Geometry: final body of the model. Coordinates: model frame, mm. A direction names the side the tool comes from. Give positions to 0.01 mm unless a question says otherwise; leave off trailing zeros. Order: outer loops, then holes, each group sorted by start corner. A loop starts at its lowest first (then second) coordinate and runs counter-clockwise, first axis right, second up. Notation, with made-up numbers: (-22.5, -21.5) -> (7.5, -21.5) arc R18 cw to (7.5, -4.5) -> close; hole circle Ø5 at (8, -23.75). An arc over 180 degrees is marked (long way). Answer in a Markdown table with one row per item. Add a question column.
Q1. Cut plane D-D on y = 0.2. Return the cut outline in (x, z) (3 decimals), and give its area (3 significant figures).
Q2. Set-up query: faces 4 (the face through (2.625, 2, -8)), 5 (the face through (4, 1, 0)), 6 (the face through (4, 2, -5.97)), 7 (the face through (4, 2, -9.27)), 8 (the face through (0, 1, -7)). Return all of +Z, -Z, +X, -X, +Y, -Y with unobstructed straight access to the full face (end or side cutting, diameter ignored); none if empty.
Q3. Contact query for flat-ended pins moving along their axis: P1, Ø0.6, axis at y = 2.5, z = -8, coming from the -X side (3 decimals); P2, Ø4, axis at x = 1, z = -3, coming from the +Y side; P3, Ø0.6, axis at x = 4.5, y = 2, coming from the +Z side; P4, Ø2, axis at x = 4.125, z = -12.045, coming from the -Y side (3 decimals). Output: stop coordinate, or through.
Q4. Pull-direction query (X, two-part tool) for faces 1 (the face through (5.625, 2, -8)), 2 (the face through (4, 1, -14.57)), 3 (the face through (3.319, 0.786, -13.096)); classes: +X half, -X half, draft (parallel to the pull), parting line (faces both ways), or undercut.
Q5. Cut plane C-C on z = -12.5. Return the cut outline in (x, y), and give its area (3 significant figures).
Q6. Cut plane A-A on z = -1.5. Return the cut outline in (x, y) (3 decimals), and give its area (4 significant figures).
Q7. Line query: line 1 along X through (y, z) = (1, -1.5) (3 decimals); line 2 along Y through (x, z) = (7.5, -1.5); line 3 along Z through (x, y) = (4.25, 1.05). Output: solid intervals per line, ascending. Write a range as from..to.
Q8. Cut plane B-B on x = 3.25. Return the cut outline in (y, z).
from build123d import *

# Parameters (mm, degrees)
SKETCH1_W                      = 8.25
SKETCH1_H                      = 14.57
BOSS_EXTRUDE1_DEPTH            = 1.55
SKETCH2_R                      = 1.325
CUT_EXTRUDE1_DEPTH             = 17.815168747
SKETCH3_W                      = 3
SKETCH3_H                      = 3.3
BOSS_EXTRUDE2_DEPTH            = 1.3
F_0_6_0_6_DIAMETER_HOLE1_D     = 0.6
F_0_6_0_6_DIAMETER_HOLE1_DEPTH = 2
F_0_6_0_6_DIAMETER_HOLE1_TIP   = 0.180258186


with BuildPart() as part:
    # Sketch1 → Boss-Extrude1 (new body)
    with BuildSketch(Plane(origin=(0, 0, 0), x_dir=(1, 0, 0), z_dir=(0, 1, 0))):
        with Locations((4.125, 7.285)):
            Rectangle(SKETCH1_W, SKETCH1_H)
    extrude(amount=BOSS_EXTRUDE1_DEPTH)

    # Sketch2 → Cut-Extrude1 (cut, through all)
    with BuildSketch(Plane(origin=(0, 1.55, 0), x_dir=(1, 0, 0), z_dir=(0, 1, 0))):
        with Locations(Location((4.125, 12.045, 0), (0, 0, 270))):
            Circle(SKETCH2_R)
    extrude(amount=-CUT_EXTRUDE1_DEPTH, mode=Mode.SUBTRACT)

    # Sketch3 → Boss-Extrude2 (add)
    with BuildSketch(Plane(origin=(0, 1.55, 0), x_dir=(1, 0, 0), z_dir=(0, 1, 0))):
        with Locations((4.125, 7.62)):
            Rectangle(SKETCH3_W, SKETCH3_H)
    extrude(amount=BOSS_EXTRUDE2_DEPTH)

    # Ø0.6 (0.6) Diameter Hole1
    with Locations(Plane(origin=(0, 1.55, 0), x_dir=(1, 0, 0), z_dir=(0, 1, 0))):
        with Locations((4.125, 1.5), (1.585, 1.5), (6.665, 1.5)):
            Hole(F_0_6_0_6_DIAMETER_HOLE1_D / 2, depth=F_0_6_0_6_DIAMETER_HOLE1_DEPTH)
            with Locations((0, 0, -(F_0_6_0_6_DIAMETER_HOLE1_DEPTH + F_0_6_0_6_DIAMETER_HOLE1_TIP / 2))):  # 118° drill point
                Cone(0, F_0_6_0_6_DIAMETER_HOLE1_D / 2, F_0_6_0_6_DIAMETER_HOLE1_TIP, mode=Mode.SUBTRACT)


solid = part.part
Completed:
| question | item | result |
|---|---|---|
| 1 | outline | (0, -14.57) -> (8.25, -14.57) -> (8.25, 0) -> (0, 0) -> close; hole circle Ø0.6 at (1.585, -1.5); hole circle Ø2.65 at (4.125, -12.045); hole circle Ø0.6 at (4.125, -1.5); hole circle Ø0.6 at (6.665, -1.5) |
| 1 | area | 114 mm² |
| 2 | face 4 | +Z, -Z, -X, +Y |
| 2 | face 5 | +Z, +X, -X, +Y, -Y |
| 2 | face 6 | +Z, +X, -X, +Y |
| 2 | face 7 | -Z, +X, -X, +Y |
| 2 | face 8 | +Z, -Z, -X, +Y, -Y |
| 3 | P1 | stops at x = 2.625 |
| 3 | P2 | stops at y = 1.55 |
| 3 | P3 | stops at z = -5.97 |
| 3 | P4 | passes through |
| 4 | face 1 | +X half |
| 4 | face 2 | draft |
| 4 | face 3 | undercut |
| 5 | outline | (0, 0) -> (2.88, 0) -> (2.88, 1.55) -> (0, 1.55) -> close; (5.37, 0) -> (8.25, 0) -> (8.25, 1.55) -> (5.37, 1.55) -> close |
| 5 | area | 8.93 mm² |
| 6 | outline | (0, 0) -> (1.285, 0) -> (1.285, 1.55) -> (0, 1.55) -> close; (1.885, 0) -> (3.825, 0) -> (3.825, 1.55) -> (1.885, 1.55) -> close; (4.425, 0) -> (6.365, 0) -> (6.365, 1.55) -> (4.425, 1.55) -> close; (6.965, 0) -> (8.25, 0) -> (8.25, 1.55) -> (6.965, 1.55) -> close |
| 6 | area | 10.00 mm² |
| 7 | line 1 | x = 0..1.285, 1.885..3.825, 4.425..6.365, 6.965..8.25 |
| 7 | line 2 | y = 0..1.55 |
| 7 | line 3 | z = -14.57..-13.36, -10.73..-1.77, -1.23..0 |
| 8 | outline | (0, -14.57) -> (1.55, -14.57) -> (1.55, -13.04) -> (0, -13.04) -> close; (0, -11.05) -> (1.55, -11.05) -> (1.55, -9.27) -> (2.85, -9.27) -> (2.85, -5.97) -> (1.55, -5.97) -> (1.55, 0) -> (0, 0) -> close |
